Model file for the job. Use its own axes, mm. Round coordinates to 2 decimals unless told otherwise and drop trailing zeros. Order: outer loops, then holes, each group sorted by start corner. A loop starts at its lowest first (then second) coordinate and runs counter-clockwise, first axis right, second up. Notation, with made-up numbers: (87.5, 26) - (99.5, 26) arc R18 cw to (99.5, 50) - close; hole circle Ø10 at (66, 50). An arc over 180 degrees is marked (long way). Answer as CSV lines item,"result". Start each with the question number.
1. Wall check: line 1 along Y through (x, z) = (0.7, 103.5); line 2 along Z through (x, y) = (2.45, 73.5); line 3 along Z through (x, y) = (1.45, 33). Give the ranges that are in metal, low to high. Write a range as [from, to].
2. Band-saw the part on A-A on z = 72. List the corners of the cut face in (x, y) (3 decimals), then the cut area to 3 significant figures.
3. Band-saw the part on C-C on z = 112.5. List the corners of the cut face in (x, y) (3 decimals).
4. Band-saw the part on B-B on x = 2. State how many separate pieces and enclosed holes the cut face has, then the cut area to 3 significant figures.
5. Pull direction Z, two halves, no side cores. Call faces 1 (the face through (1.57, 11.15, 179.01)), 2 (the face through (2, -14.858, 115)), 3 (the face through (2, 37, 202.49)): released by +Z, released by -Z, zero draft, split by the parting line, or undercut.
Autodesk Inventor part; units mm, degrees
ref_plane "YZ Plane" through (0, 0, 0) normal (1, 0, 0) x (0, 1, 0)
ref_plane "XZ Plane" through (0, 0, 0) normal (0, 1, 0) x (-1, 0, 0)
ref_plane "XY Plane" through (0, 0, 0) normal (0, 0, 1) x (1, 0, 0)
sketch "Sketch1" plane through (0, 0, 0) normal (1, 0, 0) x (0, 1, 0)
  line L0 (86.7421, 202.4896) -> (-14.8579, 202.4896)
  line L1 (-14.8579, 202.4896) -> (-14.8579, 24.6896)
  line L2 (-14.8579, 24.6896) -> (86.7421, 24.6896)
  line L3 (86.7421, 24.6896) -> (86.7421, 202.4896)
  line L4 (86.7421, 202.4896) -> (86.7421, 227.8896) construction
  point P0 (0, 0)
  dimension "d0" = 101.6
  dimension "d1" = 177.8
  dimension "d23" = 25.4
extrude "Extrusion1" add sketch "Sketch1" along normal blind 3.175
sketch "Sketch2" plane through (3.175, 0, 0) normal (1, 0, 0) x (0, 0, -1)
  line L0 (-202.4896, 86.7421) -> (-202.4896, -14.8579) construction
  line L1 (-202.4896, 35.9421) -> (-177.0896, 35.9421) construction
  line L2 (-177.0896, 35.9421) -> (-144.0696, 35.9421) construction
  circle A0 centre (-144.0696, 35.9421) radius 11.1125
  line L3 (-144.0696, 35.9421) -> (-103.4296, 35.9421) construction
  line L4 (-103.4296, 35.9421) -> (-62.7896, 35.9421) construction
  circle A1 centre (-103.4296, 35.9421) radius 11.1125
  circle A2 centre (-62.7896, 35.9421) radius 14.2875
  circle A3 centre (-177.0896, 35.9421) radius 9.525
  point P0 (0, 0)
  dimension "d4" = 25.4
  dimension "d5" = 33.02
  dimension "d7" = 22.225
  dimension "d8" = 40.64
  dimension "d9" = 40.64
  dimension "d10" = 22.225
  dimension "d11" = 28.575
  dimension "d14" = 19.05
extrude "Extrusion2" cut sketch "Sketch2" against normal blind 12.7
sketch "Sketch3" plane through (0, 0, 0) normal (-1, 0, 0) x (0, 0, 1)
  circle A0 centre (177.0896, 35.9421) radius 9.525
  circle A1 centre (177.0836, 61.3421) radius 2.0193
  circle A2 centre (177.0836, 10.5421) radius 2.0193
  line L0 (177.0836, 61.3421) -> (177.0836, 10.5421) construction
  point P0 (0, 0)
  dimension "d17" = 4.0386
  dimension "d18" = 4.0386
extrude "Extrusion3" cut sketch "Sketch3" against normal blind 25.4 contours A1 | A2
sketch "Sketch4" plane through (3.175, 0, 0) normal (1, 0, 0) x (0, 0, -1)
  line L0 (-24.6896, 86.7421) -> (-202.4896, 86.7421) construction
  line L1 (-202.4896, 86.7421) -> (-189.7896, 86.7421) construction
  line L2 (-189.7896, 86.7421) -> (-189.7896, 74.0421) construction
  line L3 (-189.7896, 74.0421) -> (-202.4896, 74.0421) construction
  line L4 (-202.4896, 74.0421) -> (-202.4896, 86.7421) construction
  line L5 (-202.4896, 86.7421) -> (-202.4896, -14.8579) construction
  line L6 (-202.4896, -14.8579) -> (-189.7896, -14.8579) construction
  line L7 (-189.7896, -14.8579) -> (-189.7896, -2.1579) construction
  line L8 (-189.7896, -2.1579) -> (-202.4896, -2.1579) construction
  line L9 (-202.4896, -2.1579) -> (-202.4896, -14.8579) construction
  line L10 (-202.4896, -14.8579) -> (-24.6896, -14.8579) construction
  line L11 (-24.6896, -14.8579) -> (-37.3896, -14.8579) construction
  line L12 (-37.3896, -14.8579) -> (-37.3896, -2.1579) construction
  line L13 (-37.3896, -2.1579) -> (-24.6896, -2.1579) construction
  line L14 (-24.6896, -2.1579) -> (-24.6896, -14.8579) construction
  line L15 (-24.6896, 86.7421) -> (-37.3896, 86.7421) construction
  line L16 (-37.3896, 86.7421) -> (-37.3896, 74.0421) construction
  line L17 (-37.3896, 74.0421) -> (-24.6896, 74.0421) construction
  line L18 (-24.6896, 74.0421) -> (-24.6896, 86.7421) construction
  circle A0 centre (-189.7896, 74.0421) radius 2.5797
  circle A1 centre (-37.3896, 74.0421) radius 2.5797
  circle A2 centre (-37.3896, -2.1579) radius 2.5797
  circle A3 centre (-189.7896, -2.1579) radius 2.5797
  point P0 (0, 0)
  dimension "d24" = 12.7
  dimension "d25" = 12.7
  dimension "d26" = 12.7
  dimension "d27" = 12.7
  dimension "d28" = 12.7
  dimension "d29" = 12.7
  dimension "d30" = 12.7
  dimension "d31" = 12.7
  dimension "d32" = 5.1594
  dimension "d33" = 5.1594
  dimension "d34" = 5.1594
  dimension "d35" = 5.1594
extrude "Extrusion4" cut sketch "Sketch4" against normal blind 25.4
properties part number "ARm Gearbox Plate"
Reply:
1,line 1,"y = [-14.86, 24.83], [47.05, 86.74]"
1,line 2,"z = [24.69, 34.87], [39.91, 187.27], [192.31, 202.49]"
1,line 3,"z = [24.69, 48.81], [76.77, 92.71], [114.15, 133.35], [154.79, 168.03], [186.15, 202.49]"
2,outline,"(0, -14.858) - (3.175, -14.858) - (3.175, 25.02) - (0, 25.02) - close; (0, 46.865) - (3.175, 46.865) - (3.175, 86.742) - (0, 86.742) - close"
2,area,"253 mm2"
3,outline,"(0, -14.858) - (3.175, -14.858) - (3.175, 29.522) - (0, 29.522) - close; (0, 42.362) - (3.175, 42.362) - (3.175, 86.742) - (0, 86.742) - close"
4,separate pieces,"1"
4,enclosed holes,"10"
4,area,"16,300 mm2"
5,face 1,"undercut"
5,face 2,"zero draft"
5,face 3,"released by +Z"
